from build123d import *

# Parameters (mm, degrees)
SKETCH1_R               = 38.1
SKETCH1_R_2             = 28.702
BOSS_EXTRUDE1_DEPTH     = 4
SKETCH2_R               = 1.5
CUT_EXTRUDE1_DEPTH      = 5
CUT_EXTRUDE2_DEPTH      = 2
CUT_EXTRUDE3_DEPTH      = 1
CUT_EXTRUDE3_DEPTH_BACK = 5


with BuildPart() as part:
    # Sketch1 → Boss-Extrude1 (new body)
    with BuildSketch(Plane.XY):
        Circle(SKETCH1_R)
        Circle(SKETCH1_R_2, mode=Mode.SUBTRACT)
    extrude(amount=BOSS_EXTRUDE1_DEPTH)

    # Sketch2 → Cut-Extrude1 (cut, through all)
    with BuildSketch(Plane.XY.offset(4)):
        with Locations((0, 35.814)):
            Circle(SKETCH2_R)
        with Locations((17.907, 31.015833811)):
            Circle(SKETCH2_R)
        with Locations((31.015833811, 17.907)):
            Circle(SKETCH2_R)
        with Locations((35.814, 0)):
            Circle(SKETCH2_R)
        with Locations((31.015833811, -17.907)):
            Circle(SKETCH2_R)
        with Locations((17.907, -31.015833811)):
            Circle(SKETCH2_R)
        with Locations((0, -35.814)):
            Circle(SKETCH2_R)
        with Locations((-17.907, -31.015833811)):
            Circle(SKETCH2_R)
        with Locations((-31.015833811, -17.907)):
            Circle(SKETCH2_R)
        with Locations((-35.814, 0)):
            Circle(SKETCH2_R)
        with Locations((-31.015833811, 17.907)):
            Circle(SKETCH2_R)
        with Locations((-17.907, 31.015833811)):
            Circle(SKETCH2_R)
    extrude(amount=-CUT_EXTRUDE1_DEPTH, mode=Mode.SUBTRACT)

    # Sketch3 → Cut-Extrude2 (cut)
    with BuildSketch(Plane.XY.offset(4)):
        Polygon((-2.9, 37.989472226), (0, 39.162631561), (2.9, 37.989472226), (2.9, 34.139684219), (0, 32.465368439), (-2.9, 34.139684219), align=None)
        Polygon((16.483262442, 34.349848024), (19.581315781, 33.915833811), (21.506209784, 31.449848024), (19.581315781, 28.115833811), (16.232684219, 28.115833811), (14.558368439, 31.015833811), align=None)
        Polygon((31.449848024, 21.506209784), (33.915833811, 19.581315781), (34.349848024, 16.483262442), (31.015833811, 14.558368439), (28.115833811, 16.232684219), (28.115833811, 19.581315781), align=None)
        Polygon((37.989472226, 2.9), (39.162631561, 0), (37.989472226, -2.9), (34.139684219, -2.9), (32.465368439, 0), (34.139684219, 2.9), align=None)
        Polygon((34.349848024, -16.483262442), (33.915833811, -19.581315781), (31.449848024, -21.506209784), (28.115833811, -19.581315781), (28.115833811, -16.232684219), (31.015833811, -14.558368439), align=None)
        Polygon((21.506209784, -31.449848024), (19.581315781, -33.915833811), (16.483262442, -34.349848024), (14.558368439, -31.015833811), (16.232684219, -28.115833811), (19.581315781, -28.115833811), align=None)
        Polygon((2.9, -37.989472226), (0, -39.162631561), (-2.9, -37.989472226), (-2.9, -34.139684219), (0, -32.465368439), (2.9, -34.139684219), align=None)
        Polygon((-16.483262442, -34.349848024), (-19.581315781, -33.915833811), (-21.506209784, -31.449848024), (-19.581315781, -28.115833811), (-16.232684219, -28.115833811), (-14.558368439, -31.015833811), align=None)
        Polygon((-31.449848024, -21.506209784), (-33.915833811, -19.581315781), (-34.349848024, -16.483262442), (-31.015833811, -14.558368439), (-28.115833811, -16.232684219), (-28.115833811, -19.581315781), align=None)
        Polygon((-37.989472226, -2.9), (-39.162631561, 0), (-37.989472226, 2.9), (-34.139684219, 2.9), (-32.465368439, 0), (-34.139684219, -2.9), align=None)
        Polygon((-34.349848024, 16.483262442), (-33.915833811, 19.581315781), (-31.449848024, 21.506209784), (-28.115833811, 19.581315781), (-28.115833811, 16.232684219), (-31.015833811, 14.558368439), align=None)
        Polygon((-21.506209784, 31.449848024), (-19.581315781, 33.915833811), (-16.483262442, 34.349848024), (-14.558368439, 31.015833811), (-16.232684219, 28.115833811), (-19.581315781, 28.115833811), align=None)
    extrude(amount=-CUT_EXTRUDE2_DEPTH, mode=Mode.SUBTRACT)

    # Sketch4 → Cut-Extrude3 (cut, two sides)
    with BuildSketch(Plane.XY.offset(4)) as cut_extrude3_sk:
        with BuildLine():
            Line((-9.861005618, 36.801773982), (9.861005618, -36.801773982))
            ThreePointArc((9.861005618, -36.801773982), (36.801773982, 9.861005618), (-9.861005618, 36.801773982))
        make_face()
    extrude(amount=CUT_EXTRUDE3_DEPTH, mode=Mode.SUBTRACT)
    extrude(cut_extrude3_sk.sketch, amount=-CUT_EXTRUDE3_DEPTH_BACK, mode=Mode.SUBTRACT)


solid = part.part
Design review of the part built by this model. Coordinates are the model's own, in mm. A direction names the side the tool comes from. Coordinates: 2 decimals unless noted, no trailing zeros. Loops run counter-clockwise (first coordinate to the right, second up) from the corner with the lowest first, then second, coordinate; pieces in that order, holes last. Notation, with made-up numbers: (75.5, -0.75) - (95.5, -0.75) arc R25 cw to (95.5, 34.25) - close; hole circle Ø1 at (52, 76). An arc over 180 degrees is marked (long way). Use CSV: the item, a comma, the result in double quotes. Start each with the question number.
1. To check wall thickness, follow probe 1 along Y at (x, z) = (-26, 1); probe 2 along Y at (x, z) = (-16, 1.05); probe 3 along X at (y, z) = (1, 1.6). State the ranges of each line that lie inside material, in increasing order.
2. For faces 4 (the flat face through (-15.38, 29.59, 3.01)), 5 (the flat face through (-27, -11, 4)), 6 (the flat face through (-29.76, -20.53, 3.01)), list the 3-axis set-ups (+Z, -Z, +X, -X, +Y, -Y) from which the entire face can be reached by the end or side of a thin tool; tool diameter is ignored.
3. Clearance check with flat-ended pins moving along their axes: pin 1 (1.5 mm diameter, centred on y = -26, z = 1, fed in from -X); pin 2 (2 mm diameter, centred on y = -35.5, z = 3, fed in from -X); pin 3 (5 mm diameter, centred on x = -31.02, y = -17.91, fed in from +Z); pin 4 (6 mm diameter, centred on x = -35.5, y = 0.5, fed in from +Z). State where each tip first meets the part, or that it passes through.
4. Mouldability with a two-part tool opening along Y and no side actions: class faces 1 (the cylindrical face through (-37.01, -9.05, 1.97)), 2 (the flat face through (-20.53, 29.76, 3.01)), 3 (the cylindrical face through (-1.19, -36.73, 1.01)) as released by +Y, released by -Y, zero draft, split by the parting line, or undercut.
5. Add section B-B on y = -7.5. Give the boundary of the cut face in (x, z).
Resolved:
1,probe 1,"-27.85 to -12.16, 12.16 to 27.85"
1,probe 2,"-34.58 to -23.83, 23.83 to 34.58"
1,probe 3,"-38.09 to -36.93, -34.7 to -28.68"
2,face 4,"+Z"
2,face 5,"+Z, +X, -X, +Y, -Y"
2,face 6,"+Z, -X"
3,pin 1,"x = -28.53"
3,pin 2,"x = -16.17"
3,pin 3,"z = 2"
3,pin 4,"z = 4"
4,face 1,"split by the parting line"
4,face 2,"released by +Y"
4,face 3,"undercut"
5,outline,"(-37.35, 0) - (-27.7, 0) - (-27.7, 4) - (-37.35, 4) - close"
